Autodesk Inventor part; units mm, degrees
ref_plane "Start Plane" through (0, 0, 0) normal (0, 0, 1) x (1, 0, 0)
ref_plane "End Plane" through (0, 0, 123.7262) normal (0, 0, 1) x (1, 0, 0)
ref_plane "Work Plane5" through (0, -10, 123.7262) normal (0, 0.3492, 0.9371) x (1, 0, 0)
ref_plane "Start Plane" through (0, 0, 0) normal (0, 0, 1) x (1, 0, 0)
ref_plane "End Plane" through (0, 0, 123.7262) normal (0, 0, 1) x (1, 0, 0)
sketch "Sketch" plane through (0, 0, 0) normal (0, 0, 1) x (1, 0, 0)
  line L0 (-10, -7) -> (-10, 7)
  line L1 (-7, 10) -> (7, 10)
  line L2 (10, 7) -> (10, -7)
  line L3 (7, -10) -> (-7, -10)
  arc A0 (-10, -7) -> (-7, -10) centre (-7, -7) ccw
  arc A1 (-7, 10) -> (-10, 7) centre (-7, 7) ccw
  arc A2 (10, 7) -> (7, 10) centre (7, 7) ccw
  arc A3 (7, -10) -> (10, -7) centre (7, -7) ccw
  arc A4 (-7, 8) -> (-8, 7) centre (-7, 7) ccw
  line L4 (-7, 8) -> (7, 8)
  arc A5 (8, 7) -> (7, 8) centre (7, 7) ccw
  line L5 (8, 7) -> (8, -7)
  arc A6 (7, -8) -> (8, -7) centre (7, -7) ccw
  line L6 (7, -8) -> (-7, -8)
  arc A7 (-8, -7) -> (-7, -8) centre (-7, -7) ccw
  line L7 (-8, -7) -> (-8, 7)
  line L8 (0, 14.8698) -> (0, -14.8698) construction
  line L9 (-14.8698, 0) -> (14.8698, 0) construction
  dimension "d7" = 3
  dimension "d10" = 20
  dimension "d11" = 20
  dimension "d12" = 2
  dimension "d15" = 10
  dimension "d16" = 10
extrude "Body" add sketch "Sketch" along normal up to surface (123.7262 mm away) from surface at 0
sketch "Sketch3" plane through (0, 0, 0) normal (0, 0, 1) x (1, 0, 0)
  line L0 (0, 0) -> (10, 0)
ref_plane "Work Plane3" through (0, 0, 0) normal (0, -1, 0) x (1, 0, 0)
sketch "Sketch4" plane through (0, 0, 0) normal (0, -1, 0) x (1, 0, 0)
  line L0 (-2, 0) -> (12, 0)
  line L1 (-2, 123.7262) -> (12, 123.7262)
  dimension "d18" = 123.7262
ref_plane "Work Plane5" through (0, -10, 123.7262) normal (0, 0.3492, 0.9371) x (1, 0, 0)
split "Split2" plane through (0, -10, 123.7262) removes the side toward (0, 0.3492, 0.9371)
sketch "Sketch5" plane through (10, -7, 0) normal (1, 0, 0) x (0, 0, -1)
  circle A0 centre (-100, 7) radius 4
  line L0 (0, 0) -> (-122.6083, 0)
  line L1 (0, 14) -> (0, 0)
  line L2 (0, 14) -> (-117.3917, 14)
  line L3 (-117.3917, 14) -> (-122.6083, 0)
  point P0 (0, 7)
extrude "Extrusion2" cut sketch "Sketch5" against normal through all contours A0
equation "\"d7\" = G_IR"
equation "\"d10\" = G_H"
equation "\"d11\" = G_W"
equation "\"d12\" = G_T"
equation "\"d15\" = 0.5 * d10"
equation "\"d16\" = 0.5 * d11"
equation "\"d3\" = G_L"
equation "\"G_W\" = 20"
equation "\"G_H\" = 20"
equation "\"G_T\" = 2"
equation "\"G_IR\" = 3"
equation "\"G_L\" = d18"
equation "\"G_OFFSET_START\" = 0"
equation "\"G_OFFSET_END\" = 3.72616"
equation "\"d14\" = G_OFFSET_END + B_L"
properties part number "ISO 12633-2 - 20x20x2 - 123,73" material "Steel, Mild"
Input: part model. Units: mm. Frame: model coordinates. A direction names the side the tool comes from. Give positions to 0.01 mm unless a question says otherwise; leave off trailing zeros. Write each loop counter-clockwise with the first axis right and the second up, starting at its lowest first coordinate (ties: lowest second). Pieces come first, ordered by that corner, then holes.
Q1. Set-up query: faces 4 (the face through (0, 8, 58)), 5 (the face through (-9.1, -9.14, 61)). Return all of +Z, -Z, +X, -X, +Y, -Y with unobstructed straight access to the full face (end or side cutting, diameter ignored); none if empty.
Q2. Material intervals for probe 1 along X at (y, z) = (-2.5, 68); probe 2 along Y at (x, z) = (-8.65, 100), sorted ascending.
Q3. Pull-direction query (Y, two-part tool) for faces 1 (the face through (-9.14, 9.1, 57.87)), 2 (the face through (-9, 0, 104)), 3 (the face through (-9, 0, 0)); classes: pulls with the +Y half, pulls with the -Y half, needs draft (parallel to the pull), parting line crosses it, or undercut.
Q4. Section A-A, the plane x = -2.25. Output: boundary loops of the cut face in (y, z), plus the area to 3 significant figures.
Q5. Section D-D, the plane z = 56.5. Output: boundary loops of the cut face in (x, y), plus the area to 3 significant figures.
Q6. Section B-B, the plane z = 100. Output: boundary loops of the cut face in (x, y), plus the area to 3 significant figures.
Q7. Section C-C, the plane y = 0. Output: boundary loops of the cut face in (x, z), plus the area to 3 significant figures.
Filled in:
1. face 4: +Z, -Z
1. face 5: +Z, -Z, -X, -Y
2. probe 1: x = -10 to -8, 8 to 10
2. probe 2: y = -9.51 to -4, 4 to 9.51
3. face 1: pulls with the +Y half
3. face 2: undercut
3. face 3: needs draft
4. outline: (-10, 0) - (-8, 0) - (-8, 122.98) - (-10, 123.73) - close; (8, 0) - (10, 0) - (10, 116.27) - (8, 117.02) - close
4. area: 480 mm2
5. outline: (-10, -7) arc R3 ccw to (-7, -10) - (7, -10) arc R3 ccw to (10, -7) - (10, 7) arc R3 ccw to (7, 10) - (-7, 10) arc R3 ccw to (-10, 7) - close; hole (-8, -7) arc R1 ccw to (-7, -8) - (7, -8) arc R1 ccw to (8, -7) - (8, 7) arc R1 ccw to (7, 8) - (-7, 8) arc R1 ccw to (-8, 7) - close
5. area: 137 mm2
6. outline: (-10, -7) arc R3 ccw to (-7, -10) - (7, -10) arc R3 ccw to (10, -7) - (10, -4) - (8, -4) - (8, -7) arc R1 cw to (7, -8) - (-7, -8) arc R1 cw to (-8, -7) - (-8, -4) - (-10, -4) - close; (-10, 4) - (-8, 4) - (-8, 7) arc R1 cw to (-7, 8) - (7, 8) arc R1 cw to (8, 7) - (8, 4) - (10, 4) - (10, 7) arc R3 ccw to (7, 10) - (-7, 10) arc R3 ccw to (-10, 7) - close
6. area: 105 mm2
7. outline: (-10, 0) - (-8, 0) - (-8, 96) - (-10, 96) - close; (-10, 104) - (-8, 104) - (-8, 120) - (-10, 120) - close; (8, 0) - (10, 0) - (10, 96) - (8, 96) - close; (8, 104) - (10, 104) - (10, 120) - (8, 120) - close
7. area: 448 mm2
